Part model, mm, in its own coordinate system. Face numbers are marked on the shaded views. A direction names the side the tool comes from. Round coordinates to 2 decimals unless told otherwise and drop trailing zeros. Write each loop counter-clockwise with the first axis right and the second up, starting at its lowest first coordinate (ties: lowest second). Pieces come first, ordered by that corner, then holes. Notation, with made-up numbers: (6, 34) -> (57, 34) arc R30 ccw to (57, 59) -> close; hole circle Ø8 at (73, 63). An arc over 180 degrees is marked (long way). Use CSV: the item, a comma, the result in double quotes. Start each with the question number.
(1) Which spindle directions (+Z, -Z, +X, -X, +Y, -Y) get a long thin tool onto all of the face, cutting with end or side? Do the marked faces 1 and 2. Say none if no direction does.
(2) Saw through at C-C (x = 11). Give the cut face in (y, z).
(3) Saw through at B-B (z = -11). Give the cut face in (x, y), plus the area to 3 significant figures.
(4) Two-plate mould, pull along Z, no slides. Class the marked faces 3, 4 and 5: released by +Z, released by -Z, zero draft, split by the parting line, or undercut.
(5) Probe line 1 (X direction, y = 5.75, z = -39); line 2 (Z direction, x = -24.5, y = 1); line 3 (X direction, y = 8, z = -3). List the from-to ranges inside material, lowest first. Write a range as [from, to].
(6) Saw through at D-D (x = 34). Give the cut face in (y, z), plus the area to 3 significant figures.
(7) Saw through at A-A (y = 8.75). Give the cut face in (x, z), plus the area to 3 significant figures.
(8) Drop flat-ended pins along their axis: pin 1 (4 mm diameter, centred on y = 4.5, z = -47.5, fed in from +X); pin 2 (4 mm diameter, centred on y = 4.5, z = -47.5, fed in from -X). Give the stop position or say it passes through.
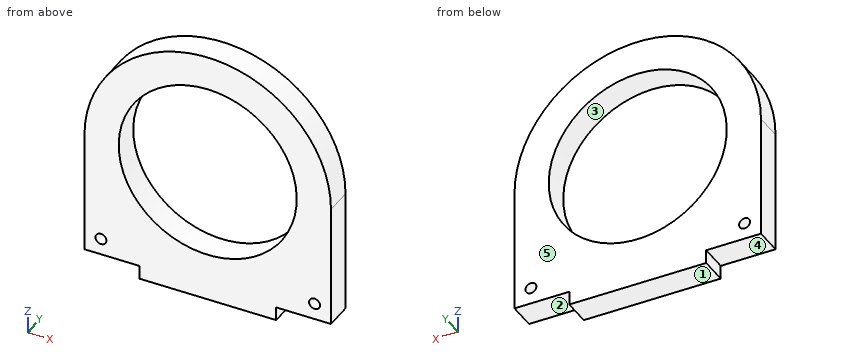
```python
from build123d import *

# Parameters (mm, degrees)
SKETCH_1_R      = 32.5
SKETCH_1_R_2    = 2
EXTRUDE_1_DEPTH = 10


with BuildPart() as part:
    # 스케치1 → 보스-돌출1 (new body)
    with BuildSketch(Plane(origin=(0, 0, 0), x_dir=(1, 0, 0), z_dir=(0, 1, 0))):
        with BuildLine():
            Line((-25, 45), (-25, 50))
            Line((-25, 50), (25, 50))
            Line((25, 50), (25, 45))
            Line((25, 45), (45, 45))
            Line((45, 45), (45, 0))
            ThreePointArc((45, 0), (0, -45), (-45, 0))
            Line((-45, 0), (-45, 45))
            Line((-45, 45), (-25, 45))
        make_face()
        with Locations(Location((0, 0, 0), (0, 0, 270))):
            Circle(SKETCH_1_R, mode=Mode.SUBTRACT)
        with Locations(Location((-39, 39, 0), (0, 0, 270))):
            Circle(SKETCH_1_R_2, mode=Mode.SUBTRACT)
        with Locations(Location((39, 39, 0), (0, 0, 270))):
            Circle(SKETCH_1_R_2, mode=Mode.SUBTRACT)
    extrude(amount=EXTRUDE_1_DEPTH)


solid = part.part
```
Answers:
1,face 1,"-Z, +X, -X, +Y, -Y"
1,face 2,"-Z, +X, +Y, -Y"
2,outline,"(0, -50) -> (10, -50) -> (10, -30.58) -> (0, -30.58) -> close; (0, 30.58) -> (10, 30.58) -> (10, 43.63) -> (0, 43.63) -> close"
3,outline,"(-45, 0) -> (-30.58, 0) -> (-30.58, 10) -> (-45, 10) -> close; (30.58, 0) -> (45, 0) -> (45, 10) -> (30.58, 10) -> close"
3,area,"288 mm²"
4,face 3,"undercut"
4,face 4,"released by -Z"
4,face 5,"zero draft"
5,line 1,"x = [-45, -41], [-37, 37], [41, 45]"
5,line 2,"z = [-50, -21.35], [21.35, 37.75]"
5,line 3,"x = [-45, -32.36], [32.36, 45]"
6,outline,"(0, -45) -> (10, -45) -> (10, 29.48) -> (0, 29.48) -> close"
6,area,"745 mm²"
7,outline,"(-45, -45) -> (-25, -45) -> (-25, -50) -> (25, -50) -> (25, -45) -> (45, -45) -> (45, 0) arc R45 ccw to (-45, 0) -> close; hole circle Ø4 at (-39, -39); hole circle Ø65 at (0, 0); hole circle Ø4 at (39, -39)"
7,area,"4,140 mm²"
8,pin 1,"stops at x = 25"
8,pin 2,"stops at x = -25"
